Work out the finished part from the listing and answer in its coordinate system (mm). Face numbers are marked on the shaded views. A direction names the side the tool comes from. Give positions to 0.01 mm unless a question says otherwise; leave off trailing zeros. Write each loop counter-clockwise with the first axis right and the second up, starting at its lowest first coordinate (ties: lowest second). Pieces come first, ordered by that corner, then holes.
1) Find section D-D (y = -18.5). Determine the outline of the cut face in (x, z), plus the area to 3 significant figures.
2) A tool of negligible diameter and unlimited length cuts with its end or side. For the marked faces 1, 2 and 3, from which of +Z, -Z, +X, -X, +Y, -Y can it reach the whole face along a straight path? Write none if from no direction.
3) Given pin 1 Ø5 at (x, y) = (10.5, 4) entering from -Z; pin 2 Ø1.4 at (y, z) = (3.5, 3.5) entering from -X; pin 3 Ø1 at (x, z) = (-16.5, 3) entering from +Y; pin 4 Ø1 at (x, z) = (17.5, -3.5) entering from +Y, each flat-ended and moving along its own axis, determine where each tip first touches the part or whether it passes through.
4) Straight lines are drawn through the part: probe 1 along Z at (x, y) = (0, -14); probe 2 along Z at (x, y) = (15.5, 10); probe 3 along X at (y, z) = (7, 2.5). For each, find the intervals that lie inside material, in ascending order.
5) Find section B-B (y = 0). Determine the outline of the cut face in (x, z).
6) Determine the mould class of the marked faces 4, 5 and 6 for opening direction X: pulls with the +X half, pulls with the -X half, needs draft (parallel to the pull), parting line crosses it, or undercut.
7) Find section A-A (z = 0). Determine the outline of the cut face in (x, y), plus the area to 3 significant figures.
8) Find section C-C (x = 0). Determine the outline of the cut face in (y, z), plus the area to 3 significant figures.
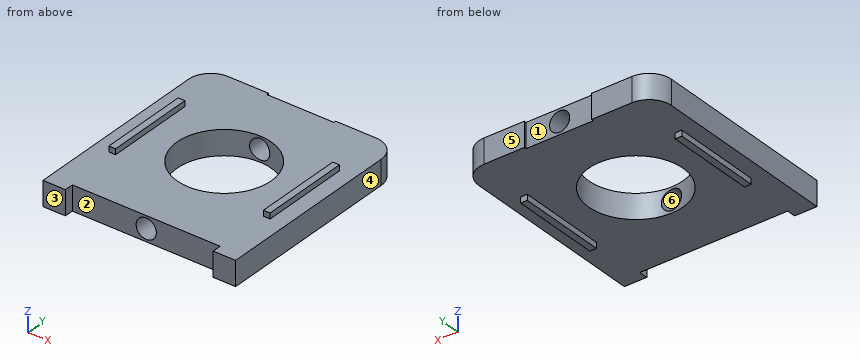
```python
from build123d import *

# Parameters (mm, degrees)
SKETCH1_W            = 43
SKETCH1_H            = 45
SKETCH1_R            = 10.5
BOSS_EXTRUDE1_DEPTH  = 2.75
FILLET1_R            = 5
SKETCH2_W            = 15
SKETCH2_H            = 0.5
CUT_EXTRUDE1_DEPTH   = 10
M4_CLEARANCE_HOLE1_D = 4.5
SKETCH5_W            = 1.5
SKETCH5_H            = 20
BOSS_EXTRUDE2_DEPTH  = 4
SKETCH6_W            = 5
SKETCH6_H            = 2
BOSS_EXTRUDE3_DEPTH  = 2.75


with BuildPart() as part:
    # Sketch1 → Boss-Extrude1 (new, symmetric)
    with BuildSketch(Plane.XY):
        Rectangle(SKETCH1_W, SKETCH1_H)
        Circle(SKETCH1_R, mode=Mode.SUBTRACT)
    extrude(amount=BOSS_EXTRUDE1_DEPTH, both=True)

    # Fillet1
    fillet1_edges = [part.edges().sort_by_distance(p)[0] for p in [
        (-21.5, 22.5, 0),
        (21.5, 22.5, 0),
    ]]
    fillet(fillet1_edges, radius=FILLET1_R)

    # Sketch2 → Cut-Extrude1 (cut)
    with BuildSketch(Plane.XY.offset(2.75)):
        with Locations((0, 22.25)):
            Rectangle(SKETCH2_W, SKETCH2_H)
    extrude(amount=-CUT_EXTRUDE1_DEPTH, mode=Mode.SUBTRACT)

    # M4 Clearance Hole1 (through all)
    with Locations(Plane(origin=(0, 22, 0), x_dir=(1, 0, 0), z_dir=(0, 1, 0))):
        with Locations((0, 0)):
            Hole(M4_CLEARANCE_HOLE1_D / 2)

    # Sketch5 → Boss-Extrude2 (add, symmetric)
    with BuildSketch(Plane.XY):
        with Locations((-17.25, 0)):
            Rectangle(SKETCH5_W, SKETCH5_H)
        with Locations((17.25, 0)):
            Rectangle(SKETCH5_W, SKETCH5_H)
    extrude(amount=BOSS_EXTRUDE2_DEPTH, both=True)

    # Sketch6 → Boss-Extrude3 (add, symmetric)
    with BuildSketch(Plane.XY):
        with Locations((-19, -23.5)):
            Rectangle(SKETCH6_W, SKETCH6_H)
        with Locations((19, -23.5)):
            Rectangle(SKETCH6_W, SKETCH6_H)
    extrude(amount=BOSS_EXTRUDE3_DEPTH, both=True)


solid = part.part
```
Results:
1. outline: (-21.5, -2.75) - (21.5, -2.75) - (21.5, 2.75) - (-21.5, 2.75) - close; hole circle Ø4.5 at (0, 0)
1. area: 221 mm2
2. face 1: +Z, -Z, +Y
2. face 2: +Z, -Z, -Y
2. face 3: +Z, -Z, +X, -X, -Y
3. pin 1: stops at z = -2.75
3. pin 2: stops at x = -18
3. pin 3: stops at y = 22.5
3. pin 4: stops at y = 10
4. probe 1: z = -2.75 to -2.25, 2.25 to 2.75
4. probe 2: z = -2.75 to 2.75
4. probe 3: x = -21.5 to -7.83, 7.83 to 21.5
5. outline: (-21.5, -2.75) - (-18, -2.75) - (-18, -4) - (-16.5, -4) - (-16.5, -2.75) - (-10.5, -2.75) - (-10.5, 2.75) - (-16.5, 2.75) - (-16.5, 4) - (-18, 4) - (-18, 2.75) - (-21.5, 2.75) - close; (10.5, -2.75) - (16.5, -2.75) - (16.5, -4) - (18, -4) - (18, -2.75) - (21.5, -2.75) - (21.5, 2.75) - (18, 2.75) - (18, 4) - (16.5, 4) - (16.5, 2.75) - (10.5, 2.75) - close
6. face 4: pulls with the +X half
6. face 5: needs draft
6. face 6: undercut
7. outline: (-21.5, -24.5) - (-16.5, -24.5) - (-16.5, -22.5) - (-2.25, -22.5) - (-2.25, -10.26) arc R10.5 cw to (-2.25, 10.26) - (-2.25, 22) - (-7.5, 22) - (-7.5, 22.5) - (-16.5, 22.5) arc R5 ccw to (-21.5, 17.5) - close; (2.25, -22.5) - (16.5, -22.5) - (16.5, -24.5) - (21.5, -24.5) - (21.5, 17.5) arc R5 ccw to (16.5, 22.5) - (7.5, 22.5) - (7.5, 22) - (2.25, 22) - (2.25, 10.26) arc R10.5 cw to (2.25, -10.26) - close
7. area: 1,480 mm2
8. outline: (-22.5, -2.75) - (-10.5, -2.75) - (-10.5, -2.25) - (-22.5, -2.25) - close; (-22.5, 2.25) - (-10.5, 2.25) - (-10.5, 2.75) - (-22.5, 2.75) - close; (10.5, -2.75) - (22, -2.75) - (22, -2.25) - (10.5, -2.25) - close; (10.5, 2.25) - (22, 2.25) - (22, 2.75) - (10.5, 2.75) - close
8. area: 23.5 mm2
